Design review of the part built by this model. Coordinates are the model's own, in mm. Round coordinates to 2 decimals unless told otherwise and drop trailing zeros. Write each loop counter-clockwise with the first axis right and the second up, starting at its lowest first coordinate (ties: lowest second). Pieces come first, ordered by that corner, then holes.
from build123d import *

# Parameters (mm, degrees)
F1_DEPTH = 5
F2_R     = 1.65
F3_DEPTH = 18.8
F4_R     = 3
F5_DEPTH = 3
F6_DEPTH = 25


with BuildPart() as f1:
    # F0 (on Top) → F1 (new body)
    with BuildSketch(Plane.XY):
        Polygon((50, 10), (50, 27.5), (-50, 27.5), (-50, 10), (-70, 10), (-70, -10), (-50, -10), (-50, -27.5), (50, -27.5), (50, -10), (70, -10), (70, 10), align=None)
    extrude(amount=F1_DEPTH)

    # F2 (on face) → F3 (cut, symmetric)
    with BuildSketch(Plane.XY.offset(5)):
        with Locations((-34.7, 24)):
            Circle(F2_R)
        with Locations((40.3, 24)):
            Circle(F2_R)
        with Locations((-36.1, -24)):
            Circle(F2_R)
        with Locations((46.6, -24)):
            Circle(F2_R)
    extrude(amount=F3_DEPTH, both=True, mode=Mode.SUBTRACT)

    # F4 (on face) → F5 (join)
    with BuildSketch(Plane.XY.offset(5)):
        with Locations((-34.7, 24)):
            Circle(F4_R)
        with Locations((40.3, 24)):
            Circle(F4_R)
        with Locations((46.6, -24)):
            Circle(F4_R)
        with Locations((-36.1, -24)):
            Circle(F4_R)
    extrude(amount=F5_DEPTH)

    # F2 (on face) → F6 (cut)
    with BuildSketch(Plane.XY.offset(5)):
        with Locations((-34.7, 24)):
            Circle(F2_R)
        with Locations((40.3, 24)):
            Circle(F2_R)
        with Locations((-36.1, -24)):
            Circle(F2_R)
        with Locations((46.6, -24)):
            Circle(F2_R)
    extrude(amount=F6_DEPTH, mode=Mode.SUBTRACT)


solid = f1.part
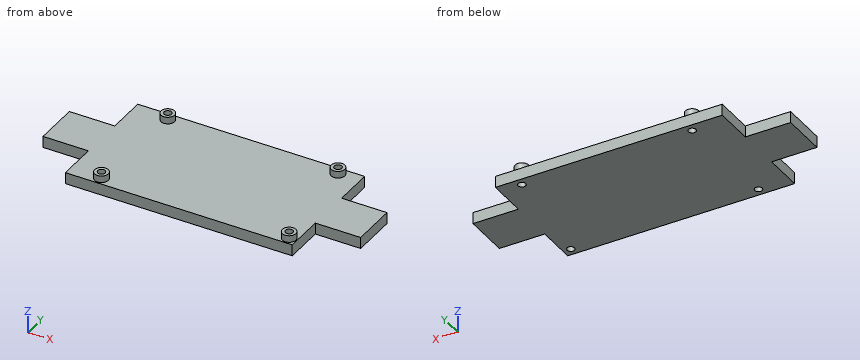
1) Add section A-A on z = 6.25. State the section outline as (x, y) points, and give its area (3 significant figures).
2) Add section B-B on x = 40.3. State the section outline as (y, z) points.
3) Add section C-C on y = -24. State the section outline as (x, z) points, and give its area (3 significant figures).
4) For line 1 along Y through (x, z) = (46.6, 2.45); line 2 along X through (y, z) = (-22.5, 7.25); line 3 along X through (y, z) = (-23, 1.5), list the stretches that pass through material, from the lowest coordinate up.
5) For P1, Ø4, axis at y = 20, z = 2.5, coming from the -X side; P2, Ø3, axis at y = 21.5, z = 3.5, coming from the +X side; P3, Ø1.5, axis at x = -58.5, z = 3.5, coming from the -Y side, all flat-tipped, find the tip position at first contact; note any pin that passes through.
6) Add section D-D on y = 5. State the section outline as (x, z) points.
Computed:
1. outline: circle Ø6 at (-36.1, -24); circle Ø6 at (-34.7, 24); circle Ø6 at (40.3, 24); circle Ø6 at (46.6, -24); hole circle Ø3.3 at (-36.1, -24); hole circle Ø3.3 at (-34.7, 24); hole circle Ø3.3 at (40.3, 24); hole circle Ø3.3 at (46.6, -24)
1. area: 78.9 mm2
2. outline: (-27.5, 0) - (22.35, 0) - (22.35, 8) - (21, 8) - (21, 5) - (-27.5, 5) - close; (25.65, 0) - (27.5, 0) - (27.5, 5) - (27, 5) - (27, 8) - (25.65, 8) - close
3. outline: (-50, 0) - (-37.75, 0) - (-37.75, 8) - (-39.1, 8) - (-39.1, 5) - (-50, 5) - close; (-34.45, 0) - (44.95, 0) - (44.95, 8) - (43.6, 8) - (43.6, 5) - (-33.1, 5) - (-33.1, 8) - (-34.45, 8) - close; (48.25, 0) - (50, 0) - (50, 5) - (49.6, 5) - (49.6, 8) - (48.25, 8) - close
3. area: 483 mm2
4. line 1: y = -27.5 to -25.65, -22.35 to 27.5
4. line 2: x = -38.7 to -36.79, -35.41 to -33.5, 44 to 45.91, 47.29 to 49.2
4. line 3: x = -50 to -37.41, -34.79 to 45.29, 47.91 to 50
5. P1: stops at x = -50
5. P2: stops at x = 50
5. P3: stops at y = -10
6. outline: (-70, 0) - (70, 0) - (70, 5) - (-70, 5) - close
